For this review, take the finished solid that the model builds, in its own axes (mm). Face numbers are marked on the shaded views. A direction names the side the tool comes from. Give positions to 0.01 mm unless a question says otherwise; leave off trailing zeros. Write each loop counter-clockwise with the first axis right and the second up, starting at its lowest first coordinate (ties: lowest second). Pieces come first, ordered by that corner, then holes.
Q1. Mouldability with a two-part tool opening along X and no side actions: class the marked faces 1, 2 and 3 as released by +X, released by -X, zero draft, split by the parting line, or undercut.
Q2. For line 1 (Y direction, x = 0, z = 6.75); line 2 (Y direction, x = -1, z = 8.5); line 3 (Z direction, x = -3.5, y = 11.5), list the stretches that pass through material, from the lowest coordinate up.
Q3. Machinability: for the marked faces 4, 5 and 6, which of the approach directions +Z, -Z, +X, -X, +Y, -Y give a long, thin tool a straight path to every point of the face, cutting with its end or side? Answer none if there is none.
Q4. We need section D-D (y = 6). Write out the cut boundary in (x, z), then the cut area to 3 significant figures.
Q5. Insertion check: P1, Ø2, axis at x = 10, y = 6.5, coming from the +Z side; P2, Ø1, axis at y = -7.5, z = 6.5, coming from the +X side; P3, Ø5, axis at x = 7.5, z = 8.5, coming from the +Y side. Each pin has a flat end and moves straight along its axis. Give the tip position at first contact, or say it passes through.
Q6. We need section A-A (y = 0). Write out the cut boundary in (x, z), then the cut area to 3 significant figures.
Q7. We need section C-C (z = 3.5). Write out the cut boundary in (x, y), then the cut area to 3 significant figures.
```python
from build123d import *

# Parameters (mm, degrees)
F0_R     = 10.4775
F1_DEPTH = 10.2743
F0_R_2   = 12.5476
F2_DEPTH = 7.6708
F3_START = 2.5019
F0_R_3   = 15.0241
F3_DEPTH = 5.1689
F4_D     = 6.0452


# Not quite as in the source:
# - a feature names something its author has since deleted; it is built from what else it names


with BuildPart() as f1:
    # F0 (on Top) → F1 (new body)
    with BuildSketch(Plane.XY):
        Circle(F0_R)
    extrude(amount=F1_DEPTH)

    # F0 (on Top) → F2 (join)
    with BuildSketch(Plane.XY):
        Circle(F0_R_2)
        Circle(F0_R, mode=Mode.SUBTRACT)
    extrude(amount=F2_DEPTH)

    # F0 (on Top) → F3 (join)
    with BuildSketch(Plane.XY.offset(F3_START)):
        Circle(F0_R_3)
        Circle(F0_R_2, mode=Mode.SUBTRACT)
    extrude(amount=F3_DEPTH)

    # F4 (through all)
    with Locations(Plane(origin=(0, 0, 0), x_dir=(1, 0, 0), z_dir=(0, 0, -1))):
        with Locations((0, 0)):
            Hole(F4_D / 2)


solid = f1.part
```
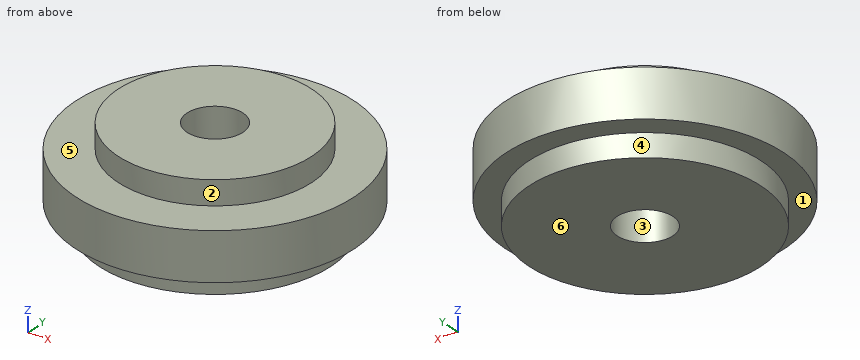
Computed:
1. face 1: zero draft
1. face 2: split by the parting line
1. face 3: undercut
2. line 1: y = -15.02 to -3.02, 3.02 to 15.02
2. line 2: y = -10.43 to -2.85, 2.85 to 10.43
2. line 3: z = 0 to 7.67
3. face 4: -Z
3. face 5: +Z
3. face 6: -Z, +X, -X, +Y, -Y
4. outline: (-13.77, 2.5) - (-11.02, 2.5) - (-11.02, 0) - (11.02, 0) - (11.02, 2.5) - (13.77, 2.5) - (13.77, 7.67) - (8.59, 7.67) - (8.59, 10.27) - (-8.59, 10.27) - (-8.59, 7.67) - (-13.77, 7.67) - close
4. area: 242 mm2
5. P1: stops at z = 7.67
5. P2: stops at x = 13.29
5. P3: stops at y = 14.12
6. outline: (-15.02, 2.5) - (-12.55, 2.5) - (-12.55, 0) - (-3.02, 0) - (-3.02, 10.27) - (-10.48, 10.27) - (-10.48, 7.67) - (-15.02, 7.67) - close; (3.02, 0) - (12.55, 0) - (12.55, 2.5) - (15.02, 2.5) - (15.02, 7.67) - (10.48, 7.67) - (10.48, 10.27) - (3.02, 10.27) - close
6. area: 211 mm2
7. outline: circle Ø30.05 at (0, 0); hole circle Ø6.05 at (0, 0)
7. area: 680 mm2
